```python
from build123d import *

# Parameters (mm, degrees)
SKETCH2_R           = 6
BOSS_EXTRUDE2_DEPTH = 5
SKETCH4_R           = 15
BOSS_EXTRUDE3_DEPTH = 40
BOSS_EXTRUDE4_START = -40
BOSS_EXTRUDE4_DEPTH = 40
CHAMFER1_SIZE       = 0.5
CHAMFER2_SIZE       = 0.5


with BuildPart() as part:
    # Sketch2 → Boss-Extrude2 (new body)
    with BuildSketch(Plane(origin=(0, 0, 0), x_dir=(1, 0, 0), z_dir=(0, 1, 0))):
        with Locations(Location((0, 0, 0), (0, 0, 270))):
            Circle(SKETCH2_R)
    extrude(amount=BOSS_EXTRUDE2_DEPTH)

    # Sketch4 → Boss-Extrude3 (add)
    with BuildSketch(Plane(origin=(0, 5, 0), x_dir=(1, 0, 0), z_dir=(0, 1, 0))):
        with Locations(Location((0, 0, 0), (0, 0, 270))):
            Circle(SKETCH4_R)
    extrude(amount=BOSS_EXTRUDE3_DEPTH)

    # Sketch5 → Boss-Extrude4 (add)
    with BuildSketch(Plane(origin=(0, 45, 0), x_dir=(1, 0, 0), z_dir=(0, 1, 0)).offset(BOSS_EXTRUDE4_START)):
        with BuildLine():
            ThreePointArc((-11.802749471, 9.257165059), (-10.606601718, 10.606601718), (-9.257165059, 11.802749471))
            ThreePointArc((-9.257165059, 11.802749471), (-10.686189168, 12.11373051), (-12.015763486, 12.722870267))
            Line((-12.015763486, 12.722870267), (-12.722870267, 12.015763486))
            ThreePointArc((-12.722870267, 12.015763486), (-12.11373051, 10.686189168), (-11.802749471, 9.257165059))
        make_face()
        with BuildLine():
            ThreePointArc((-1.8, 14.891608375), (-0.901630293, 14.972877573), (0, 15))
            Line((0, 15), (0, 17.492855685))
            Line((0, 17.492855685), (-0.5, 17.492855685))
            ThreePointArc((-0.5, 17.492855685), (-1.009424163, 16.121977815), (-1.8, 14.891608375))
        make_face()
        with BuildLine():
            Line((0, 17.492855685), (0, 15))
            ThreePointArc((0, 15), (0.901630293, 14.972877573), (1.8, 14.891608375))
            ThreePointArc((1.8, 14.891608375), (1.009424163, 16.121977815), (0.5, 17.492855685))
            Line((0.5, 17.492855685), (0, 17.492855685))
        make_face()
        with BuildLine():
            ThreePointArc((12.015763486, 12.722870267), (10.686189168, 12.11373051), (9.257165059, 11.802749471))
            ThreePointArc((9.257165059, 11.802749471), (10.606601718, 10.606601718), (11.802749471, 9.257165059))
            ThreePointArc((11.802749471, 9.257165059), (12.11373051, 10.686189168), (12.722870267, 12.015763486))
            Line((12.722870267, 12.015763486), (12.015763486, 12.722870267))
        make_face()
        with BuildLine():
            ThreePointArc((-14.891608375, -1.8), (-15, 0), (-14.891608375, 1.8))
            ThreePointArc((-14.891608375, 1.8), (-16.121977815, 1.009424163), (-17.492855685, 0.5))
            Line((-17.492855685, 0.5), (-17.492855685, -0.5))
            ThreePointArc((-17.492855685, -0.5), (-16.121977815, -1.009424163), (-14.891608375, -1.8))
        make_face()
        with BuildLine():
            ThreePointArc((-9.257165059, -11.802749471), (-10.606601718, -10.606601718), (-11.802749471, -9.257165059))
            ThreePointArc((-11.802749471, -9.257165059), (-12.11373051, -10.686189168), (-12.722870267, -12.015763486))
            Line((-12.722870267, -12.015763486), (-12.015763486, -12.722870267))
            ThreePointArc((-12.015763486, -12.722870267), (-10.686189168, -12.11373051), (-9.257165059, -11.802749471))
        make_face()
        with BuildLine():
            ThreePointArc((1.8, -14.891608375), (0, -15), (-1.8, -14.891608375))
            ThreePointArc((-1.8, -14.891608375), (-1.009424163, -16.121977815), (-0.5, -17.492855685))
            Line((-0.5, -17.492855685), (0.5, -17.492855685))
            ThreePointArc((0.5, -17.492855685), (1.009424163, -16.121977815), (1.8, -14.891608375))
        make_face()
        with BuildLine():
            Line((12.015763486, -12.722870267), (12.722870267, -12.015763486))
            ThreePointArc((12.722870267, -12.015763486), (12.11373051, -10.686189168), (11.802749471, -9.257165059))
            ThreePointArc((11.802749471, -9.257165059), (10.606601718, -10.606601718), (9.257165059, -11.802749471))
            ThreePointArc((9.257165059, -11.802749471), (10.686189168, -12.11373051), (12.015763486, -12.722870267))
        make_face()
        with BuildLine():
            ThreePointArc((17.492855685, 0.5), (16.121977815, 1.009424163), (14.891608375, 1.8))
            ThreePointArc((14.891608375, 1.8), (14.972877573, 0.901630293), (15, 0))
            ThreePointArc((15, 0), (14.972877573, -0.901630293), (14.891608375, -1.8))
            ThreePointArc((14.891608375, -1.8), (16.121977815, -1.009424163), (17.492855685, -0.5))
            Line((17.492855685, -0.5), (17.492855685, 0.5))
        make_face()
    extrude(amount=BOSS_EXTRUDE4_DEPTH)

    # Chamfer1
    chamfer1_edges = [part.edges().sort_by_distance(p)[0] for p in [
        (0, 0, -6),
    ]]
    chamfer(chamfer1_edges, length=CHAMFER1_SIZE)

    # Chamfer2
    chamfer2_edges = [part.edges().sort_by_distance(p)[0] for p in [
        (-13.858192988, 5, -5.740251485),
        (-5.740251485, 5, -13.858192988),
        (5.740251485, 5, -13.858192988),
        (-13.858192988, 5, 5.740251485),
        (-5.740251485, 5, 13.858192988),
        (5.740251485, 5, 13.858192988),
        (13.858192988, 5, 5.740251485),
        (13.858192988, 5, -5.740251485),
    ]]
    chamfer(chamfer2_edges, length=CHAMFER2_SIZE)


solid = part.part
```
Model file for the job. Use its own axes, mm. A direction names the side the tool comes from. Coordinates: 2 decimals unless noted, no trailing zeros. Order: outer loops, then holes, each group sorted by start corner. A loop starts at its lowest first (then second) coordinate and runs counter-clockwise, first axis right, second up. Notation, with made-up numbers: (71.5, 15.25) -> (95.5, 15.25) arc R28 ccw to (95.5, 35.25) -> close; hole circle Ø3 at (-9, -22). An arc over 180 degrees is marked (long way). Answer as a JSON object with one key per item and string values. Group by question number.
1) Drill centre lines: L1, parallel to X at y = 17, z = -12.5; L2, parallel to Z at x = -4.5, y = 7. Where is each one in solid material? Low to high.
2) Pull direction X, two halves, no side cores. Call faces 4 (the face through (16.16, 24.72, -0.99)), 5 (the face through (-5.573, 5.198, -13.6)), 6 (the face through (5.69, 24.97, 13.88)), 7 (the face through (-1.01, 24.72, 16.12)): +X half, -X half, draft (parallel to the pull), parting line (faces both ways), or undercut.
3) Flat gauge pins, fed straight in: pin 1 (8 mm diameter, centred on x = -12, z = 1, fed in from -Y); pin 2 (12 mm diameter, centred on x = 9.5, y = 29.5, fed in from -Z); pin 3 (12 mm diameter, centred on x = 12, y = 21, fed in from +Z). Where does each tip first touch, or does it go through?
4) Which spindle directions (+Z, -Z, +X, -X, +Y, -Y) get a long thin tool onto all of the face, cutting with end or side? Do faces 1 (the face through (-13.836, 24.974, -5.793)), 2 (the face through (-5.68, 5.2, 13.56)), 3 (the face through (13.56, 5.2, 5.68)). Say none if no direction does.
5) Cut at B-B, the plane z = -11. Write the cut outline in (x, y).
6) Cut at C-C, the plane z = 10.5. Write the cut outline in (x, y).
Check values:
{
 "1": {"L1": "x = -12.24 to -11.61, -8.29 to 8.29, 11.61 to 12.24", "L2": "z = -14.31 to 14.31"},
 "2": {"face 4": "+X half", "face 5": "undercut", "face 6": "undercut", "face 7": "-X half"},
 "3": {"pin 1": "stops at y = 5", "pin 2": "stops at z = -14.59", "pin 3": "stops at z = 13.75"},
 "4": {"face 1": "-X, +Y, -Y", "face 2": "+Z, -Y", "face 3": "+X, -Y"},
 "5": {"outline": "(-12.23, 5) -> (12.23, 5) -> (12.23, 45) -> (-12.23, 45) -> close"},
 "6": {"outline": "(-12.05, 5) -> (12.05, 5) -> (12.05, 45) -> (-12.05, 45) -> close"}
}
